from build123d import *

# Parameters (mm, degrees)
SKETCH1_R            = 60.7
BOSS_EXTRUDE1_DEPTH  = 1.5
M6_CLEARANCE_HOLE1_D = 6.6
CIRPATTERN2_COUNT    = 4


with BuildPart() as part:
    # Sketch1 → Boss-Extrude1 (new, symmetric)
    with BuildSketch(Plane(origin=(0, 0, 0), x_dir=(1, 0, 0), z_dir=(0, 1, 0))):
        with Locations(Location((0, 0, 0), (0, 0, 270))):
            Circle(SKETCH1_R)
    extrude(amount=BOSS_EXTRUDE1_DEPTH, both=True)

    # M6 Clearance Hole1 (through all)
    with Locations(Plane(origin=(0, 1.5, 0), x_dir=(1, 0, 0), z_dir=(0, 1, 0))):
        with Locations((50.7, 0)):
            m6_clearance_hole1 = Hole(M6_CLEARANCE_HOLE1_D / 2)

    # CirPattern2: M6 Clearance Hole1 ×4 about axis
    cirpattern2_axis = Axis((0, 0, 0), (0, 1, 0))
    for i in range(1, CIRPATTERN2_COUNT):
        add(m6_clearance_hole1.rotate(cirpattern2_axis, i * 360 / CIRPATTERN2_COUNT), mode=Mode.SUBTRACT)


solid = part.part
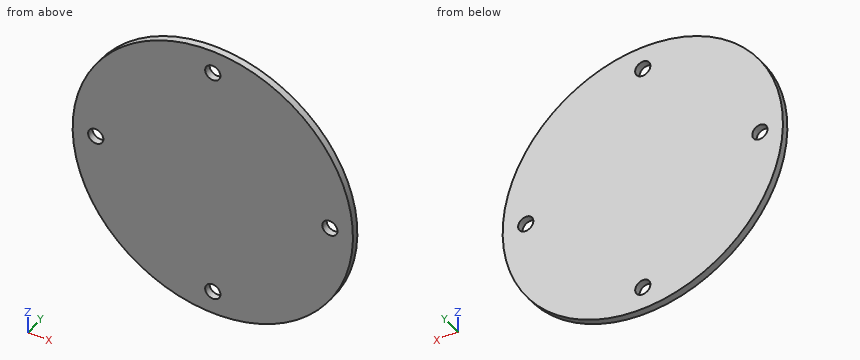
Read the model definition and answer for the solid it produces. Units are mm, in the model's axes. Coordinates: 2 decimals unless noted, no trailing zeros. Loops run counter-clockwise (first coordinate to the right, second up) from the corner with the lowest first, then second, coordinate; pieces in that order, holes last.
Q1. The part is cut by section C-C on y = -0.2. Write down the section's boundary in (x, z).
Q2. The part is cut by section B-B on z = 0. Write down the section's boundary in (x, y).
Q3. Each of these flat-tipped pins is pushed along its axis until it touches: pin 1 Ø5.5 at (x, z) = (0, 50.7) entering from +Y; pin 2 Ø1 at (x, y) = (-13.5, 1) entering from -Z; pin 3 Ø1.5 at (x, y) = (-29, 0) entering from +Z; pin 4 Ø1.5 at (x, y) = (1, 0) entering from -Z. Where does it stop, or does it pass through?
Q4. The part is cut by section A-A on x = 0. Write down the section's boundary in (y, z), and give its area (3 significant figures).
Q5. Consider probe 1 along X at (y, z) = (-0.1, 52); probe 2 along Z at (x, y) = (50.7, 0.85); probe 3 along X at (y, z) = (0.9, 50.5). Determine where each line is inside the solid, lowest interval first.
Q6. The part is cut by section D-D on x = 51. Write down the section's boundary in (y, z).
Results below:
1. outline: circle Ø121.4 at (0, 0); hole circle Ø6.6 at (-50.7, 0); hole circle Ø6.6 at (0, -50.7); hole circle Ø6.6 at (0, 50.7); hole circle Ø6.6 at (50.7, 0)
2. outline: (-60.7, -1.5) - (-54, -1.5) - (-54, 1.5) - (-60.7, 1.5) - close; (-47.4, -1.5) - (47.4, -1.5) - (47.4, 1.5) - (-47.4, 1.5) - close; (54, -1.5) - (60.7, -1.5) - (60.7, 1.5) - (54, 1.5) - close
3. pin 1: passes through
3. pin 2: stops at z = -59.29
3. pin 3: stops at z = 53.73
3. pin 4: stops at z = -60.7
4. outline: (-1.5, -60.7) - (1.5, -60.7) - (1.5, -54) - (-1.5, -54) - close; (-1.5, -47.4) - (1.5, -47.4) - (1.5, 47.4) - (-1.5, 47.4) - close; (-1.5, 54) - (1.5, 54) - (1.5, 60.7) - (-1.5, 60.7) - close
4. area: 325 mm2
5. probe 1: x = -31.31 to -3.03, 3.03 to 31.31
5. probe 2: z = -33.38 to -3.3, 3.3 to 33.38
5. probe 3: x = -33.68 to -3.29, 3.29 to 33.68
6. outline: (-1.5, -32.92) - (1.5, -32.92) - (1.5, -3.29) - (-1.5, -3.29) - close; (-1.5, 3.29) - (1.5, 3.29) - (1.5, 32.92) - (-1.5, 32.92) - close
